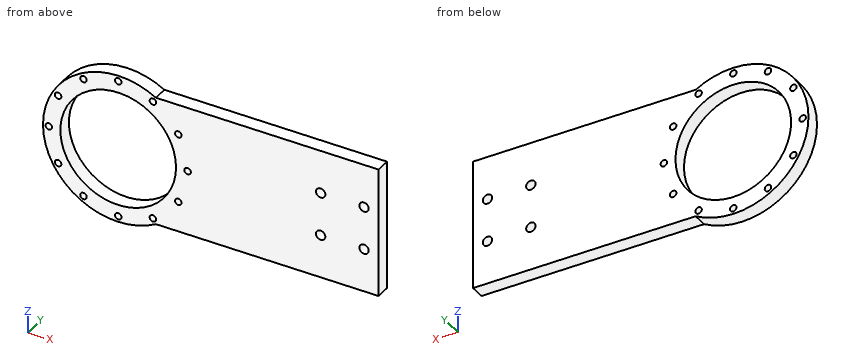
from build123d import *

# Parameters (mm, degrees)
SKETCH1_R            = 52
BOSS_EXTRUDE1_DEPTH  = 10
SKETCH2_W            = 180
SKETCH2_H            = 90
BOSS_EXTRUDE2_DEPTH  = 10
SKETCH3_R            = 40
CUT_EXTRUDE1_DEPTH   = 10
SKETCH4_R            = 2.25
CUT_EXTRUDE2_DEPTH   = 11
CIRPATTERN1_COUNT    = 12
SKETCH5_R            = 3.25
CUT_EXTRUDE3_DEPTH   = 11
LPATTERN1_COUNT      = 2
LPATTERN1_PITCH      = 30
LPATTERN1_COUNT_DIR2 = 2
LPATTERN1_PITCH_DIR2 = 30


with BuildPart() as part:
    # Sketch1 → Boss-Extrude1 (new body)
    with BuildSketch(Plane(origin=(0, 0, 0), x_dir=(1, 0, 0), z_dir=(0, 1, 0))):
        Circle(SKETCH1_R)
    extrude(amount=BOSS_EXTRUDE1_DEPTH)

    # Sketch2 → Boss-Extrude2 (add)
    with BuildSketch(Plane(origin=(0, 0, 0), x_dir=(1, 0, 0), z_dir=(0, 1, 0))):
        with Locations((90, 0)):
            Rectangle(SKETCH2_W, SKETCH2_H)
    extrude(amount=BOSS_EXTRUDE2_DEPTH)

    # Sketch3 → Cut-Extrude1 (cut)
    with BuildSketch(Plane(origin=(0, 10, 0), x_dir=(1, 0, 0), z_dir=(0, 1, 0))):
        Circle(SKETCH3_R)
    extrude(amount=-CUT_EXTRUDE1_DEPTH, mode=Mode.SUBTRACT)

    # Sketch4 → Cut-Extrude2 (cut, through all)
    with BuildSketch(Plane(origin=(0, 10, 0), x_dir=(1, 0, 0), z_dir=(0, 1, 0))):
        with Locations((0, 48)):
            Circle(SKETCH4_R)
    cut_extrude2 = extrude(amount=-CUT_EXTRUDE2_DEPTH, mode=Mode.SUBTRACT)

    # CirPattern1: Cut-Extrude2 ×12 about axis
    cirpattern1_axis = Axis((0, 0, 0), (0, 1, 0))
    for i in range(1, CIRPATTERN1_COUNT):
        add(cut_extrude2.rotate(cirpattern1_axis, i * 360 / CIRPATTERN1_COUNT), mode=Mode.SUBTRACT)

    # Sketch5 → Cut-Extrude3 (cut, through all)
    with BuildSketch(Plane(origin=(0, 10, 0), x_dir=(1, 0, 0), z_dir=(0, 1, 0))):
        with Locations((170, 15)):
            Circle(SKETCH5_R)
    cut_extrude3 = extrude(amount=-CUT_EXTRUDE3_DEPTH, mode=Mode.SUBTRACT)

    # LPattern1: Cut-Extrude3 2 × 2
    with Locations(*[(-i * LPATTERN1_PITCH, 0, j * LPATTERN1_PITCH_DIR2) for i in range(LPATTERN1_COUNT) for j in range(LPATTERN1_COUNT_DIR2) if (i, j) != (0, 0)]):
        add(cut_extrude3, mode=Mode.SUBTRACT)


solid = part.part
Read the model definition and answer for the solid it produces. Units are mm, in the model's axes. Coordinates: 2 decimals unless noted, no trailing zeros. Loops run counter-clockwise (first coordinate to the right, second up) from the corner with the lowest first, then second, coordinate; pieces in that order, holes last. Notation, with made-up numbers: (36, 38.25) - (49, 38.25) arc R22 cw to (49, 62.25) - close; hole circle Ø8 at (53, -25.5). An arc over 180 degrees is marked (long way). Answer in a Markdown table with one row per item.
Q1. Find section A-A on x = 140. Write down the section's boundary in (y, z).
Here are the results:
| item | result |
|---|---|
| outline | (0, -45) - (10, -45) - (10, -18.25) - (0, -18.25) - close; (0, -11.75) - (10, -11.75) - (10, 11.75) - (0, 11.75) - close; (0, 18.25) - (10, 18.25) - (10, 45) - (0, 45) - close |
Q2. Find section B-B on z = 48. Write down the section's boundary in (x, y), plus the area to 3 significant figures.
Here are the results:
| item | result |
|---|---|
| outline | (-20, 0) - (-2.25, 0) - (-2.25, 10) - (-20, 10) - close; (2.25, 0) - (20, 0) - (20, 10) - (2.25, 10) - close |
| area | 355 mm^2 |
Q3. Find section D-D on z = 0. Write down the section's boundary in (x, y).
Here are the results:
| item | result |
|---|---|
| outline | (-52, 0) - (-50.25, 0) - (-50.25, 10) - (-52, 10) - close; (-45.75, 0) - (-40, 0) - (-40, 10) - (-45.75, 10) - close; (40, 0) - (45.75, 0) - (45.75, 10) - (40, 10) - close; (50.25, 0) - (180, 0) - (180, 10) - (50.25, 10) - close |
Q4. Given P1, Ø2.5, axis at x = 0, z = 48, coming from the -Y side; P2, Ø2, axis at x = 75, y = 1, coming from the -Z side; P3, Ø6, axis at x = 11, y = 8, coming from the +Z side; P4, Ø6, axis at x = 81, y = 8, coming from the +Z side, each flat-ended and moving along its own axis, determine where each tip first touches the part or whether it passes through.
Here are the results:
| item | result |
|---|---|
| P1 | passes through |
| P2 | stops at z = -45 |
| P3 | stops at z = 51.38 |
| P4 | stops at z = 45 |
Q5. Find section C-C on x = -48. Write down the section's boundary in (y, z).
Here are the results:
| item | result |
|---|---|
| outline | (0, -20) - (10, -20) - (10, -2.25) - (0, -2.25) - close; (0, 2.25) - (10, 2.25) - (10, 20) - (0, 20) - close |
Q6. Straight lines are drawn through the part: line 1 along X through (y, z) = (7, -24.5); line 2 along X through (y, z) = (9, 22); line 3 along X through (y, z) = (4.75, -42.5). For each, find the intervals that lie inside material, in ascending order. Write a range as [from, to].
Here are the results:
| item | result |
|---|---|
| line 1 | x = [-45.87, -43.76], [-39.38, -31.62], [31.62, 39.38], [43.76, 180] |
| line 2 | x = [-47.12, -42.6], [-40.54, -33.41], [33.41, 40.54], [42.6, 180] |
| line 3 | x = [-29.96, -26.05], [-21.95, 21.95], [26.05, 180] |
